The model under review builds one solid part; all positions refer to its coordinate system, in mm. Face numbers are marked on the shaded views. A direction names the side the tool comes from. Give positions to 0.01 mm unless a question says otherwise; leave off trailing zeros. Write each loop counter-clockwise with the first axis right and the second up, starting at its lowest first coordinate (ties: lowest second). Pieces come first, ordered by that corner, then holes. Notation, with made-up numbers: (38.5, -10) -> (92.5, -10) arc R24 cw to (92.5, 29) -> close; hole circle Ø5 at (6, 77.25). An arc over 180 degrees is marked (long way). Use CSV: the item, a comma, the result in double quotes.
```python
from build123d import *

# Parameters (mm, degrees)
BOSS_EXTRUDE2_DEPTH  = 12
SKETCH4_OUTSIDE_W    = 92.038
SKETCH4_OUTSIDE_H    = 86.932
SKETCH4_OUTSIDE_R    = 16.5
CUT_EXTRUDE6_DEPTH   = 12
CUT_EXTRUDE6_DRAFT   = -60
SKETCH5_OUTSIDE_W    = 92.038
SKETCH5_OUTSIDE_H    = 86.932
SKETCH5_OUTSIDE_R    = 16.5
CUT_EXTRUDE7_DEPTH   = 12
CUT_EXTRUDE7_DRAFT   = -60
FILLET1_R            = 2.5
SKETCH9_R            = 12.5
BOSS_EXTRUDE6_DEPTH  = 5
SKETCH11_R           = 10
BOSS_EXTRUDE8_DEPTH  = 15
CHAMFER1_SIZE        = 1
FILLET2_R            = 0.5
SKETCH12_R           = 2.6
BOSS_EXTRUDE9_DEPTH  = 12
SKETCH13_R           = 2.5
BOSS_EXTRUDE10_DEPTH = 11


with BuildPart() as part:
    # Sketch3 → Boss-Extrude2 (new body)
    with BuildSketch(Plane(origin=(0, 0, 0), x_dir=(1, 0, 0), z_dir=(0, 1, 0))):
        Polygon((19.052558883, 0), (9.526279442, 16.5), (-9.526279442, 16.5), (-19.052558883, 0), (-9.526279442, -16.5), (9.526279442, -16.5), align=None)
    extrude(amount=BOSS_EXTRUDE2_DEPTH)


with BuildPart() as cut_extrude6_tool:
    # Sketch4 outside → Cut-Extrude6 (with draft: the straight prism first)
    with BuildSketch(Plane(origin=(0, 12, 0), x_dir=(1, 0, 0), z_dir=(0, 1, 0))):
        Rectangle(SKETCH4_OUTSIDE_W, SKETCH4_OUTSIDE_H)
        Circle(SKETCH4_OUTSIDE_R, mode=Mode.SUBTRACT)
    extrude(amount=-CUT_EXTRUDE6_DEPTH)
    # Cut-Extrude6: the draft: its side faces are tilted about the plane it starts from
    cut_extrude6_sides = [cut_extrude6_tool.faces().sort_by_distance(p)[0] for p in [
        (0, 6, 43.466),
        (46.019, 6, 0),
        (0, 6, -43.466),
        (-46.019, 6, 0),
        (-16.5, 6, 0),
    ]]
    draft(cut_extrude6_sides, Plane(origin=(0, 12, 0), x_dir=(1, 0, 0), z_dir=(0, 1, 0)), CUT_EXTRUDE6_DRAFT)


with BuildPart() as part_1:
    add(part.part)

    # Cut-Extrude6: cut by cut_extrude6_tool
    add(cut_extrude6_tool.part, mode=Mode.SUBTRACT)


with BuildPart() as cut_extrude7_tool:
    # Sketch5 outside → Cut-Extrude7 (with draft: the straight prism first)
    with BuildSketch(Plane.XZ):
        Rectangle(SKETCH5_OUTSIDE_W, SKETCH5_OUTSIDE_H)
        Circle(SKETCH5_OUTSIDE_R, mode=Mode.SUBTRACT)
    extrude(amount=-CUT_EXTRUDE7_DEPTH)
    # Cut-Extrude7: the draft: its side faces are tilted about the plane it starts from
    cut_extrude7_sides = [cut_extrude7_tool.faces().sort_by_distance(p)[0] for p in [
        (0, 6, -43.466),
        (46.019, 6, 0),
        (0, 6, 43.466),
        (-46.019, 6, 0),
        (-16.5, 6, 0),
    ]]
    draft(cut_extrude7_sides, Plane.XZ, CUT_EXTRUDE7_DRAFT)


with BuildPart() as part_2:
    add(part_1.part)

    # Cut-Extrude7: cut by cut_extrude7_tool
    add(cut_extrude7_tool.part, mode=Mode.SUBTRACT)

    # Fillet1
    fillet1_edges = [part_2.edges().sort_by_distance(p)[0] for p in [
        (-19.052558883, 6, 0),
        (-9.526279442, 6, -16.5),
        (9.526279442, 6, -16.5),
        (19.052558883, 6, 0),
        (-9.526279442, 6, 16.5),
        (9.526279442, 6, 16.5),
    ]]
    fillet(fillet1_edges, radius=FILLET1_R)

    # Sketch9 → Boss-Extrude6 (add)
    with BuildSketch(Plane.XZ):
        with Locations(Location((0, 0, 0), (0, 0, 90))):
            Circle(SKETCH9_R)
    extrude(amount=BOSS_EXTRUDE6_DEPTH)

    # Sketch11 → Boss-Extrude8 (add)
    with BuildSketch(Plane.XZ.offset(5)):
        with Locations(Location((0, 0, 0), (0, 0, 270))):
            Circle(SKETCH11_R)
    extrude(amount=BOSS_EXTRUDE8_DEPTH)

    # Chamfer1
    chamfer1_edges = [part_2.edges().sort_by_distance(p)[0] for p in [
        (0, -20, 10),
    ]]
    chamfer(chamfer1_edges, length=CHAMFER1_SIZE)

    # Fillet2
    fillet2_edges = [part_2.edges().sort_by_distance(p)[0] for p in [
        (0, 0, -12.5),
        (0, -5, -12.5),
    ]]
    fillet(fillet2_edges, radius=FILLET2_R)

    # Sketch12 → Boss-Extrude9 (add)
    with BuildSketch(Plane.XZ.offset(20)):
        with Locations(Location((0, 0, 0), (0, 0, 270))):
            Circle(SKETCH12_R)
    extrude(amount=BOSS_EXTRUDE9_DEPTH)

    # Sketch13 → Boss-Extrude10 (add)
    with BuildSketch(Plane.XZ.offset(32)):
        with Locations(Location((0, 0, 0), (0, 0, 270))):
            Circle(SKETCH13_R)
    extrude(amount=BOSS_EXTRUDE10_DEPTH)


solid = part_2.part
```
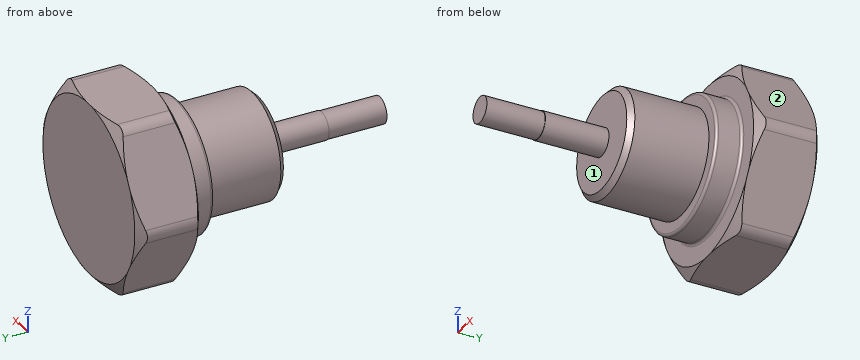
Q1. Consider section B-B (y = -22). Write out the cut boundary in (x, z), then the cut area to 3 significant figures.
Derived:
outline,"circle Ø5.2 at (0, 0)"
area,"21.2 mm2"
Q2. Consider section C-C (y = -10.5). Write out the cut boundary in (x, z), then the cut area to 3 significant figures.
Derived:
outline,"circle Ø20 at (0, 0)"
area,"314 mm2"
Q3. To check wall thickness, follow probe 1 along Y at (x, z) = (6.5, 4.5); probe 2 along Y at (x, z) = (-10, -2.5); probe 3 along Z at (x, y) = (0.5, -10). State the ranges of each line that lie inside material, in increasing order.
Derived:
probe 1,"y = -20 to 12"
probe 2,"y = -5 to 12"
probe 3,"z = -9.99 to 9.99"
Q4. Machinability: for the marked faces 1 and 2, which of the approach directions +Z, -Z, +X, -X, +Y, -Y give a long, thin tool a straight path to every point of the face, cutting with its end or side? Answer none if there is none.
Derived:
face 1,"-Y"
face 2,"+Z, +X, +Y, -Y"
Q5. Insertion check: pin 1 (1 mm diameter, centred on x = -6.5, y = -3.5, fed in from +Z); pin 2 (6 mm diameter, centred on x = -5.5, y = -10.5, fed in from -Z); pin 3 (5 mm diameter, centred on y = -31.5, z = 2.5, fed in from +X). Each pin has a flat end and moves straight along its axis. Give the tip position at first contact, or say it passes through.
Derived:
pin 1,"stops at z = 10.97"
pin 2,"stops at z = -9.68"
pin 3,"stops at x = 2.6"
